Geometry: final body of the model. Coordinates: model frame, mm. Face numbers are marked on the shaded views. A direction names the side the tool comes from. Give positions to 0.01 mm unless a question says otherwise; leave off trailing zeros. Loops run counter-clockwise (first coordinate to the right, second up) from the corner with the lowest first, then second, coordinate; pieces in that order, holes last.
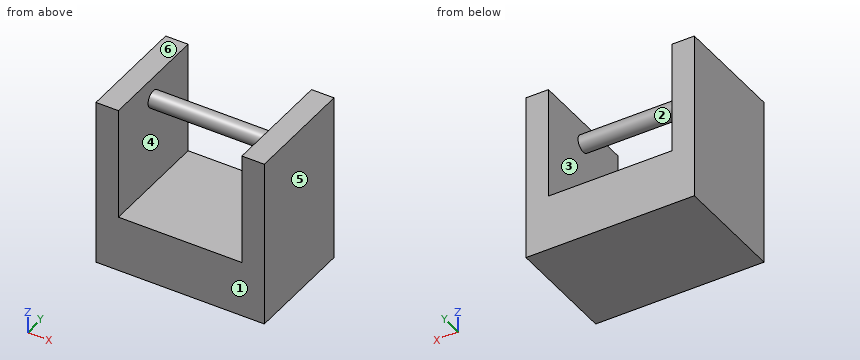
Autodesk Inventor part; units mm, degrees
ref_plane "YZ Plane" through (0, 0, 0) normal (1, 0, 0) x (0, 1, 0)
ref_plane "XZ Plane" through (0, 0, 0) normal (0, 1, 0) x (-1, 0, 0)
ref_plane "XY Plane" through (0, 0, 0) normal (0, 0, 1) x (1, 0, 0)
sketch "스케치1" plane through (0, 0, 0) normal (0, 0, 1) x (1, 0, 0)
  line L0 (0, 0) -> (150, 0)
  line L1 (150, 0) -> (150, -100)
  line L2 (150, -100) -> (0, -100)
  line L3 (0, -100) -> (0, 0)
  dimension "d0" = 150
  dimension "d1" = 100
extrude "돌출1" add sketch "스케치1" along normal blind 50
sketch "스케치2" plane through (0, 0, 50) normal (0, 0, 1) x (1, 0, 0)
  line L0 (0, -100) -> (150, -100)
  line L1 (150, -100) -> (150, 0)
  line L2 (150, 0) -> (0, 0)
  line L3 (0, 0) -> (0, -100)
  line L4 (20, 0) -> (20, -100)
  line L5 (130, 0) -> (130, -100)
  dimension "d4" = 20
  dimension "d5" = 20
extrude "돌출2" add sketch "스케치2" along normal blind 100 contours L3 L2 L4 L0 | L5 L2 L1 L0
sketch "스케치3" plane through (20, -100, 50) normal (1, 0, 0) x (0, 0, -1)
  line L0 (0, 100) -> (0, 0)
  line L1 (0, 100) -> (-100, 100)
  line L2 (-100, 0) -> (-100, 100)
  line L3 (0, 0) -> (-100, 0)
  circle A0 centre (-80, 50) radius 7.5
  point P0 (50, 100)
  dimension "d8" = 15
  dimension "d9" = 20
  dimension "d10" = 50
extrude "돌출3" add sketch "스케치3" along normal up to surface (110 mm away) contours A0
properties part number "lever1"
Item 1: Section query C-C on y = -50. Return loops of the section in (x, z).
Values follow:
outline: (0, 0) - (150, 0) - (150, 150) - (130, 150) - (130, 137.5) - (20, 137.5) - (20, 150) - (0, 150) - close; hole (20, 50) - (130, 50) - (130, 122.5) - (20, 122.5) - close
Item 2: Section query A-A on z = 69. Return loops of the section in (x, y).
Values follow:
outline: (0, -100) - (20, -100) - (20, 0) - (0, 0) - close; (130, -100) - (150, -100) - (150, 0) - (130, 0) - close
Item 3: Draft query along X for the marked faces 3, 4, 5 and 6. Return one class per face: +X half, -X half, draft (parallel to the pull), parting line (faces both ways), or undercut.
Values follow:
face 3: undercut
face 4: undercut
face 5: +X half
face 6: draft
Item 4: Pin query (flat end, axial travel): pin 1 (10 mm diameter, centred on x = 47.5, y = -70, fed in from -Z). Return the tip coordinate at first contact, or that it passes through.
Values follow:
pin 1: stops at z = 0
Item 5: Section query B-B on x = 109. Return loops of the section in (y, z).
Values follow:
outline: (-100, 0) - (0, 0) - (0, 50) - (-100, 50) - close; circle Ø15 at (-50, 130)
Item 6: Section query D-D on y = -24. Return loops of the section in (x, z).
Values follow:
outline: (0, 0) - (150, 0) - (150, 150) - (130, 150) - (130, 50) - (20, 50) - (20, 150) - (0, 150) - close
Item 7: Ray query, probe 1 along X at (y, z) = (-84.5, 83); probe 2 along Z at (x, y) = (77.5, -33); probe 3 along Z at (x, y) = (104, -52). Return the intervals inside material, ascending.
Values follow:
probe 1: x = 0 to 20, 130 to 150
probe 2: z = 0 to 50
probe 3: z = 0 to 50, 122.77 to 137.23
Item 8: Set-up query: the marked faces 1 and 2. Return all of +Z, -Z, +X, -X, +Y, -Y with unobstructed straight access to the full face (end or side cutting, diameter ignored); none if empty.
Values follow:
face 1: +Z, -Z, +X, -X, -Y
face 2: none
